Source: CAD feature listing. Evaluate the final solid. Frame: model axes, mm. Face numbers are marked on the shaded views. A direction names the side the tool comes from. Coordinates: 2 decimals unless noted, no trailing zeros. Loops run counter-clockwise (first coordinate to the right, second up) from the corner with the lowest first, then second, coordinate; pieces in that order, holes last. Notation, with made-up numbers: (60.25, 0) - (102.25, 0) arc R26 ccw to (102.25, 22) - close; hole circle Ø6 at (-12.5, 15). An arc over 180 degrees is marked (long way). Write item = value, one per line. Start each with the question number.
from build123d import *

# Parameters (mm, degrees)
F3_DEPTH = 50
F4_R     = 5


# Not quite as in the source:
# - a pattern or mirror of a feature is missing from the dataset's text; its kind, count and spacing are read off the source's solid


with BuildPart() as f1:
    # F0 (on Right) → F1 (revolve)
    with BuildSketch(Plane.YZ):
        Polygon((-300, 50), (-300, 0), (300, 0), (300, 50), (200, 50), (200, 55), (150, 55), (150, 50), (50, 50), (50, 60), (-50, 60), (-50, 50), (-150, 50), (-150, 55), (-200, 55), (-200, 50), align=None)
    revolve(axis=Axis((0, 0, 0), (0, 1, 0)))

    # F2 (on face) → F3 (cut)
    with BuildSketch(Plane.XZ.offset(300)):
        with BuildLine():
            Line((-7.5, 41.4342998332), (7.5, 41.4342998332))
            Line((7.5, 41.4342998332), (7.5, 49.4342998332))
            ThreePointArc((7.5, 49.4342998332), (0, 50), (-7.5, 49.4342998332))
            Line((-7.5, 49.4342998332), (-7.5, 41.4342998332))
        make_face()
    f3 = extrude(amount=-F3_DEPTH, mode=Mode.SUBTRACT)

    # F3_copies: F3 across plane
    add(f3.mirror(Plane.ZX), mode=Mode.SUBTRACT)

    # F4
    f4_edges = [f1.edges().sort_by_distance(p)[0] for p in [
        (-7.5, -250, 45.4343),
        (7.5, -250, 45.4343),
        (7.5, 250, 45.4343),
        (-7.5, 250, 45.4343),
    ]]
    fillet(f4_edges, radius=F4_R)


solid = f1.part
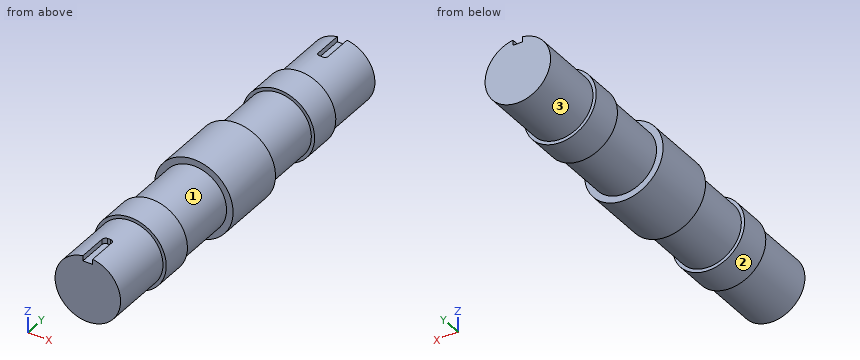
Item 1: First-contact query: pin 1 (9 mm diameter, centred on y = 280, z = 43.5, fed in from +X); pin 2 (16.5 mm diameter, centred on x = -2.5, y = -281, fed in from +Z); pin 3 (5 mm diameter, centred on y = 206.5, z = -34, fed in from -X). Flat tips, straight axial feed; report the tip coordinate or a pass-through.
Item 2: Cut plane B-B (x = 21). Return the cut outline in (y, z).
Item 3: Cut plane D-D (y = -174). Return the cut outline in (x, z).
Item 4: Cut plane C-C (y = 14). Return the cut outline in (x, z), then the cut area to 3 significant figures.
Item 5: Cut plane A-A (z = 0). Return the cut outline in (x, y).
Item 6: Reachability of the marked faces 1, 2 and 3 from +Z, -Z, +X, -X, +Y, -Y: full face, straight path, thin tool, end or side. Return the list, or none.
Item 7: Material intervals for L1, parallel to Z at x = -1, y = -218; L2, parallel to Y at x = -23, z = 52.5; L3, parallel to Z at x = -23.5, y = 174, sorted ascending. Write a range as [from, to].
Responses:
q1.pin_1 = 31.29
q1.pin_2 = 49.43
q1.pin_3 = -38.83
q2.outline = (-300, -45.38) - (-200, -45.38) - (-200, -50.83) - (-150, -50.83) - (-150, -45.38) - (-50, -45.38) - (-50, -56.2) - (50, -56.2) - (50, -45.38) - (150, -45.38) - (150, -50.83) - (200, -50.83) - (200, -45.38) - (300, -45.38) - (300, 45.38) - (200, 45.38) - (200, 50.83) - (150, 50.83) - (150, 45.38) - (50, 45.38) - (50, 56.2) - (-50, 56.2) - (-50, 45.38) - (-150, 45.38) - (-150, 50.83) - (-200, 50.83) - (-200, 45.38) - (-300, 45.38) - close
q3.outline = circle Ø110 at (0, 0)
q4.outline = circle Ø120 at (0, 0)
q4.area = 11,300 mm2
q5.outline = (-60, -50) - (-50, -50) - (-50, -150) - (-55, -150) - (-55, -200) - (-50, -200) - (-50, -300) - (50, -300) - (50, -200) - (55, -200) - (55, -150) - (50, -150) - (50, -50) - (60, -50) - (60, 50) - (50, 50) - (50, 150) - (55, 150) - (55, 200) - (50, 200) - (50, 300) - (-50, 300) - (-50, 200) - (-55, 200) - (-55, 150) - (-50, 150) - (-50, 50) - (-60, 50) - close
q6.face_1 = none
q6.face_2 = -Y
q6.face_3 = +Y
q7.L1 = [-49.99, 49.99]
q7.L2 = [-50, 50]
q7.L3 = [-49.73, 49.73]
